```python
from build123d import *

# Parameters (mm, degrees)
IZIM1_R                     = 2.5
Y_KSEKLIK_EKSTR_ZYON1_DEPTH = 1
SCALE1_SCALE                = 0.5


with BuildPart() as part:
    # Çizim1 → Yükseklik-Ekstrüzyon1 (new body)
    with BuildSketch(Plane.XY):
        with BuildLine():
            Line((-23.446136356, -44.161959762), (-25.73775467, -42.866863479))
            Line((-25.73775467, -42.866863479), (-26.834295942, -39.938466016))
            ThreePointArc((-26.834295942, -39.938466016), (-28.201527977, -38.125336415), (-30.335428898, -37.348658075))
            Line((-30.335428898, -37.348658075), (-33.334907776, -37.164700371))
            Line((-33.334907776, -37.164700371), (-33.842709051, -34.202800331))
            ThreePointArc((-33.842709051, -34.202800331), (-34.84597704, -32.165592505), (-36.7965457, -31.002818113))
            Line((-36.7965457, -31.002818113), (-39.708425324, -30.260072511))
            Line((-39.708425324, -30.260072511), (-39.652227319, -27.255483394))
            ThreePointArc((-39.652227319, -27.255483394), (-40.255989993, -25.066366444), (-41.954126526, -23.558687864))
            Line((-41.954126526, -23.558687864), (-44.675252109, -22.283466496))
            Line((-44.675252109, -22.283466496), (-44.057045667, -19.342627369))
            ThreePointArc((-44.057045667, -19.342627369), (-44.239914432, -17.079151855), (-45.625461503, -15.279979352))
            Line((-45.625461503, -15.279979352), (-48.059435816, -13.517457571))
            Line((-48.059435816, -13.517457571), (-46.901121207, -10.744549126))
            ThreePointArc((-46.901121207, -10.744549126), (-46.656617846, -8.486899797), (-47.680491761, -6.459969953))
            Line((-47.680491761, -6.459969953), (-49.741090048, -4.272585973))
            Line((-49.741090048, -4.272585973), (-48.083701146, -1.765839874))
            ThreePointArc((-48.083701146, -1.765839874), (-47.420487313, 0.406004917), (-48.046416828, 2.588887101))
            Line((-48.046416828, 2.588887101), (-49.660641368, 5.123644113))
            Line((-49.660641368, 5.123644113), (-47.562892001, 7.275425136))
            ThreePointArc((-47.562892001, 7.275425136), (-46.504462376, 9.284526705), (-46.710273625, 11.546031539))
            Line((-46.710273625, 11.546031539), (-47.82093971, 14.338366552))
            Line((-47.82093971, 14.338366552), (-45.357143694, 16.058954583))
            ThreePointArc((-45.357143694, 16.058954583), (-43.940993675, 17.834139505), (-43.719395692, 20.094152054))
            Line((-43.719395692, 20.094152054), (-44.287157421, 23.045145208))
            Line((-44.287157421, 23.045145208), (-41.54459596, 24.273587558))
            ThreePointArc((-41.54459596, 24.273587558), (-39.820893366, 25.751969023), (-39.17973637, 27.930427214))
            Line((-39.17973637, 27.930427214), (-39.184480502, 30.935538106))
            Line((-39.184480502, 30.935538106), (-36.260310201, 31.628316593))
            ThreePointArc((-36.260310201, 31.628316593), (-34.290118058, 32.757522199), (-33.252115355, 34.777253066))
            Line((-33.252115355, 34.777253066), (-32.693673826, 37.730024144))
            Line((-32.693673826, 37.730024144), (-29.691484877, 37.862596744))
            ThreePointArc((-29.691484877, 37.862596744), (-27.544598222, 38.602623821), (-26.146521576, 40.39207739))
            Line((-26.146521576, 40.39207739), (-25, 43.301270189))
            ThreePointArc((-25, 43.301270189), (-24.226890609, 43.73851588), (-23.446136356, 44.161959762))
            ThreePointArc((-23.446136356, 44.161959762), (-21.212806241, 47.755648425), (-21.906244367, 51.929556087))
            ThreePointArc((-21.906244367, 51.929556087), (-24.232021318, 53.76021953), (-27.179564099, 53.490852446))
            ThreePointArc((-27.179564099, 53.490852446), (-59.999999835, 0.004450967), (-27.1875, -53.486819346))
            Line((-27.1875, -53.486819346), (-27.179564099, -53.490852446))
            ThreePointArc((-27.179564099, -53.490852446), (-24.232021318, -53.76021953), (-21.906244367, -51.929556087))
            ThreePointArc((-21.906244367, -51.929556087), (-21.212806241, -47.755648425), (-23.446136356, -44.161959762))
        make_face()
        with Locations((-31.620079453, -45.001895242)):
            Circle(IZIM1_R, mode=Mode.SUBTRACT)
        with Locations((-55, 0)):
            Circle(IZIM1_R, mode=Mode.SUBTRACT)
        with Locations((-28.000624989, 47.338831842)):
            Circle(IZIM1_R, mode=Mode.SUBTRACT)
    extrude(amount=Y_KSEKLIK_EKSTR_ZYON1_DEPTH)


with BuildPart() as part_1:
    # Scale1: scaled about (-43.563815172, 0.008171627, 0.5)
    add(part.part.scale(SCALE1_SCALE).moved(Location((-21.781907586, 0.004085814, 0.25))))


solid = part_1.part
```
Design review of the part built by this model. Coordinates are the model's own, in mm. A direction names the side the tool comes from. Coordinates: 2 decimals unless noted, no trailing zeros. Write each loop counter-clockwise with the first axis right and the second up, starting at its lowest first coordinate (ties: lowest second). Pieces come first, ordered by that corner, then holes.
1) Add section C-C (y = -6). Write out the cut boundary in (x, z).
2) Mouldability with a two-part tool opening along X and no side actions: class faces 3 (the flat face through (-47, 0, 0.75)), 4 (the cylindrical face through (-38.94, 16.37, 0.5)), 5 (the cylindrical face through (-38.51, -21.65, 0.5)) as +X half, -X half, draft (parallel to the pull), parting line (faces both ways), or undercut.
3) To check wall thickness, follow L1, parallel to Y at x = -35.75, z = 0.45; L2, parallel to Y at x = -46.5, z = 0.4; L3, parallel to Y at x = -39, z = 0.5. State the ranges of each line that lie inside material, in increasing order.
4) Add section B-B (z = 0.55). State how many separate pieces and enclosed holes the cut face has, plus the area to 3 significant figures.
5) Machinability: for faces 1 (the flat face through (-45.085, 7.597, 0.496)), 2 (the cylindrical face through (-33.918, -26.882, 0.496)), which of the approach directions +Z, -Z, +X, -X, +Y, -Y give a long, thin tool a straight path to every point of the face, cutting with its end or side? Answer none if there is none.
6) Add section A-A (y = 23). Write out the cut boundary in (x, z).
Check result:
1. outline: (-51.17, 0.25) - (-45.5, 0.25) - (-45.5, 0.75) - (-51.17, 0.75) - close
2. face 3: draft
2. face 4: +X half
2. face 5: undercut
3. L1: y = -26.55 to -19.17, 19.18 to 22.42, 24.92 to 26.55
3. L2: y = -17 to -2.29, -1.9 to 2.39, 2.68 to 17
3. L3: y = -24.56 to -16.34, 16.31 to 24.57
4. separate pieces: 1
4. enclosed holes: 3
4. area: 345 mm2
5. face 1: +Z, -Z, +X
5. face 2: +Z, -Z, -Y
6. outline: (-41.05, 0.25) - (-36.84, 0.25) - (-36.84, 0.75) - (-41.05, 0.75) - close; (-34.73, 0.25) - (-32.71, 0.25) - (-32.71, 0.75) - (-34.73, 0.75) - close
